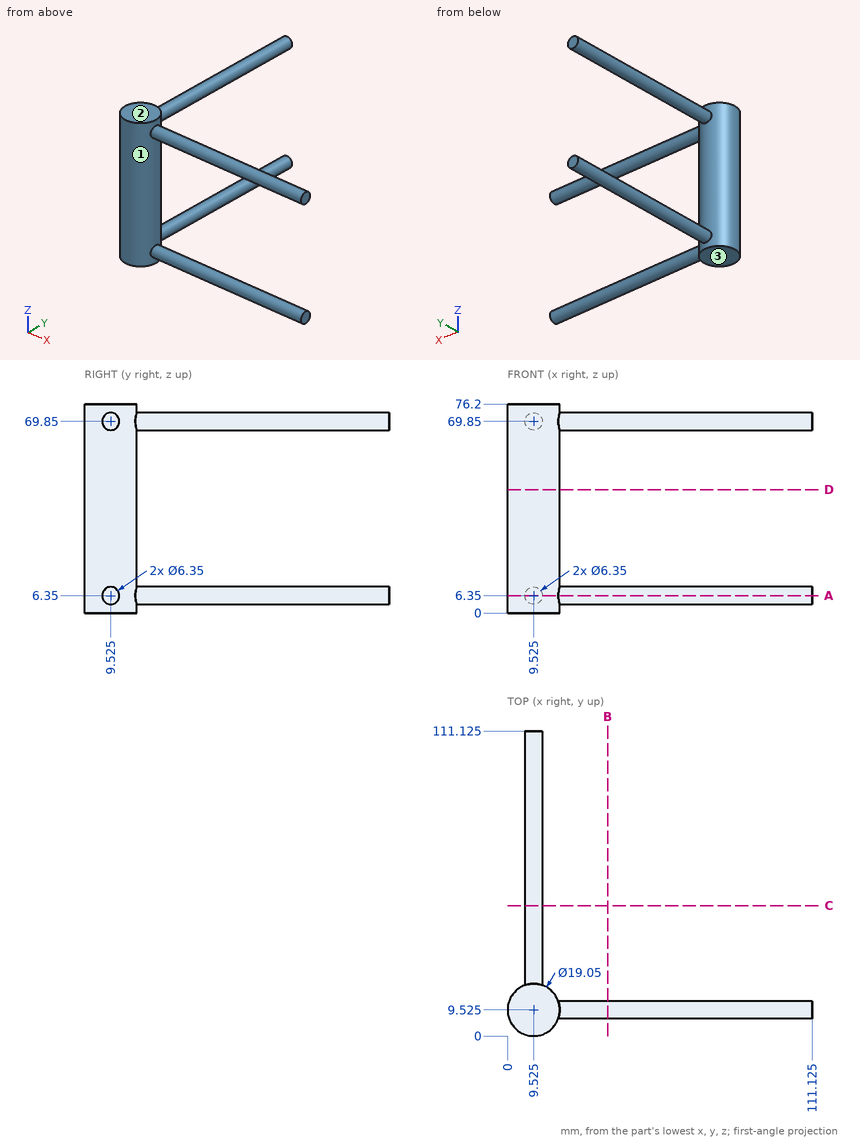
For this review, use the dimensioned drawing (mm, ordinates from the lowest corner) and the shaded views. Give positions to 0.01 mm unless a question says otherwise; leave off trailing zeros. Write each loop counter-clockwise with the first axis right and the second up, starting at its lowest first coordinate (ties: lowest second). Pieces come first, ordered by that corner, then holes.
(1) Consider section A-A, the plane z = 6.35. Give the boundary of the cut face in (x, y) (3 decimals), and give its area (3 significant figures).
(2) To check wall thickness, follow L1, parallel to Y at x = 15.5, z = 25.5; L2, parallel to X at y = 16, z = 54.5; L3, parallel to X at y = 11.5, z = 47.5. State the ranges of each line that lie inside material, in increasing order.
(3) Consider section B-B, the plane x = 36.5. Give the boundary of the cut face in (y, z) (3 decimals), and give its area (3 significant figures).
(4) The part is to be moulded in two halves that separate along Z. For the marked faces 1, 2 and 3, say which applies: released by +Z, released by -Z, zero draft, split by the parting line, or undercut.
(5) Consider section D-D, the plane z = 45. Give the boundary of the cut face in (x, y) (3 decimals).
Returned:
1. outline: (6.35, 18.505) arc R9.525 ccw (long way) to (18.505, 6.35) - (111.125, 6.35) - (111.125, 12.7) - (18.505, 12.7) arc R9.525 ccw to (12.7, 18.505) - (12.7, 111.125) - (6.35, 111.125) - close
1. area: 1,460 mm2
2. L1: y = 2.11 to 16.94
2. L2: x = 2.54 to 16.51
2. L3: x = 0.21 to 18.84
3. outline: circle Ø6.35 at (9.525, 6.35); circle Ø6.35 at (9.525, 69.85)
3. area: 63.3 mm2
4. face 1: undercut
4. face 2: released by +Z
4. face 3: released by -Z
5. outline: circle Ø19.05 at (9.525, 9.525)
